The model under review builds one solid part; all positions refer to its coordinate system, in mm. A direction names the side the tool comes from. Give positions to 0.01 mm unless a question says otherwise; leave off trailing zeros. Write each loop counter-clockwise with the first axis right and the second up, starting at its lowest first coordinate (ties: lowest second). Pieces come first, ordered by that corner, then holes. Notation, with made-up numbers: (-39, -12.5) - (4, -12.5) arc R25 cw to (4, 19.5) - close; hole circle Ø11 at (26, 9.25). An arc over 180 degrees is marked (long way). Write item = value, one per line.
```python
from build123d import *

# Parameters (mm, degrees)
SKETCH1_R           = 1.6
SKETCH1_R_2         = 1.75
SKETCH1_R_3         = 3.95
SKETCH1_R_4         = 12
BOSS_EXTRUDE1_DEPTH = 3


with BuildPart() as part:
    # Sketch1 → Boss-Extrude1 (new body)
    with BuildSketch(Plane(origin=(0, 0, 0), x_dir=(1, 0, 0), z_dir=(0, 1, 0))):
        with BuildLine():
            Line((312.373352996, 1022.190294437), (327.907309833, 1022.190294437))
            ThreePointArc((327.907309833, 1022.190294437), (328.157309833, 1022.257281735), (328.340322535, 1022.440294437))
            ThreePointArc((328.340322535, 1022.440294437), (329.126888323, 1022.543848684), (329.023336329, 1021.757282599))
            ThreePointArc((329.023336329, 1021.757282599), (328.840324865, 1021.574270305), (328.773337833, 1021.324271437))
            Line((328.773337833, 1021.324271437), (328.773337833, 1019.690242437))
            ThreePointArc((328.773337833, 1019.690242437), (328.919784442, 1019.336689047), (329.273337833, 1019.190242437))
            Line((329.273337833, 1019.190242437), (334.273335833, 1019.190242437))
            ThreePointArc((334.273335833, 1019.190242437), (334.626889492, 1019.336688397), (334.773336751, 1019.690241519))
            Line((334.773336751, 1019.690241519), (334.773336751, 1021.324268519))
            ThreePointArc((334.773336751, 1021.324268519), (334.706349307, 1021.57426848), (334.523336498, 1021.757281075))
            ThreePointArc((334.523336498, 1021.757281075), (334.419781792, 1022.543846802), (335.206347937, 1022.440295269))
            ThreePointArc((335.206347937, 1022.440295269), (335.389360338, 1022.257283911), (335.639359245, 1022.190297025))
            Line((335.639359245, 1022.190297025), (340.773337745, 1022.190297025))
            Line((340.773337745, 1022.190297025), (340.773337745, 1024.990297025))
            Line((340.773337745, 1024.990297025), (339.423337745, 1024.990297025))
            Line((339.423337745, 1024.990297025), (339.423337745, 1029.190297025))
            Line((339.423337745, 1029.190297025), (340.773337745, 1029.190297025))
            Line((340.773337745, 1029.190297025), (340.773337745, 1032.190297025))
            Line((340.773337745, 1032.190297025), (343.973337745, 1032.190297025))
            Line((343.973337745, 1032.190297025), (343.973337745, 1029.190297025))
            Line((343.973337745, 1029.190297025), (345.323337745, 1029.190297025))
            Line((345.323337745, 1029.190297025), (345.323337745, 1024.990292188))
            Line((345.323337745, 1024.990292188), (343.973337745, 1024.990292188))
            Line((343.973337745, 1024.990292188), (343.973337745, 1022.190292188))
            Line((343.973337745, 1022.190292188), (349.107314245, 1022.190292188))
            ThreePointArc((349.107314245, 1022.190292188), (349.357314245, 1022.257279486), (349.540326947, 1022.440292188))
            ThreePointArc((349.540326947, 1022.440292188), (350.326891976, 1022.543845827), (350.223341741, 1021.75728035))
            ThreePointArc((350.223341741, 1021.75728035), (350.040330277, 1021.574268055), (349.973343245, 1021.324269188))
            Line((349.973343245, 1021.324269188), (349.973343245, 1019.690240188))
            ThreePointArc((349.973343245, 1019.690240188), (350.119789854, 1019.336686797), (350.473343245, 1019.190240188))
            Line((350.473343245, 1019.190240188), (355.473340245, 1019.190240188))
            ThreePointArc((355.473340245, 1019.190240188), (355.826893904, 1019.336686148), (355.973341163, 1019.69023927))
            Line((355.973341163, 1019.69023927), (355.973341163, 1021.32426627))
            ThreePointArc((355.973341163, 1021.32426627), (355.906353816, 1021.574266257), (355.723341079, 1021.757278924))
            ThreePointArc((355.723341079, 1021.757278924), (355.619786681, 1022.543844692), (356.406352785, 1022.44029285))
            ThreePointArc((356.406352785, 1022.44029285), (356.589365548, 1022.257281171), (356.839364996, 1022.190294437))
            Line((356.839364996, 1022.190294437), (372.373340046, 1022.190294437))
            Line((372.373340046, 1022.190294437), (372.373340046, 1072.190301225))
            ThreePointArc((372.373340046, 1072.190301225), (370.908875012, 1075.72583207), (367.373345046, 1077.190299225))
            Line((367.373345046, 1077.190299225), (317.373348046, 1077.190299225))
            ThreePointArc((317.373348046, 1077.190299225), (313.837816014, 1075.725834155), (312.373352996, 1072.190301275))
            Line((312.373352996, 1072.190301275), (312.373352996, 1022.190294437))
        make_face()
        with Locations((366.893344996, 1047.842461747)):
            Circle(SKETCH1_R, mode=Mode.SUBTRACT)
        with Locations((357.873345496, 1071.990299275)):
            Circle(SKETCH1_R_2, mode=Mode.SUBTRACT)
        with Locations((357.873345496, 1040.990299275)):
            Circle(SKETCH1_R_2, mode=Mode.SUBTRACT)
        with Locations((325.373345996, 1051.490299275)):
            Circle(SKETCH1_R_3, mode=Mode.SUBTRACT)
        with Locations((342.373345496, 1056.490299275)):
            Circle(SKETCH1_R_4, mode=Mode.SUBTRACT)
        with Locations((326.873345496, 1071.990299275)):
            Circle(SKETCH1_R_2, mode=Mode.SUBTRACT)
        with Locations((326.873345496, 1040.990299275)):
            Circle(SKETCH1_R_2, mode=Mode.SUBTRACT)
        with Locations((317.853347996, 1047.84952041)):
            Circle(SKETCH1_R, mode=Mode.SUBTRACT)
        with BuildLine():
            Line((365.243389653, 1060.95296097), (365.243389653, 1056.48501097))
            ThreePointArc((365.243389653, 1056.48501097), (365.176400533, 1056.235010504), (364.993385671, 1056.051998658))
            ThreePointArc((364.993385671, 1056.051998658), (364.889836092, 1055.26543287), (365.676401176, 1055.368987799))
            ThreePointArc((365.676401176, 1055.368987799), (365.859413353, 1055.55200075), (366.109412996, 1055.618988627))
            Line((366.109412996, 1055.618988627), (367.677282996, 1055.618988627))
            ThreePointArc((367.677282996, 1055.618988627), (367.927282247, 1055.552001761), (368.110294834, 1055.368990124))
            ThreePointArc((368.110294834, 1055.368990124), (368.896860423, 1055.26543905), (368.793306996, 1056.052004329))
            ThreePointArc((368.793306996, 1056.052004329), (368.610294145, 1056.235017289), (368.543306996, 1056.485017627))
            Line((368.543306996, 1056.485017627), (368.543306996, 1060.952967627))
            ThreePointArc((368.543306996, 1060.952967627), (368.610293862, 1061.202966879), (368.793305499, 1061.385979465))
            ThreePointArc((368.793305499, 1061.385979465), (368.89685718, 1062.172545813), (368.110291294, 1062.068990627))
            ThreePointArc((368.110291294, 1062.068990627), (367.927278767, 1061.885978026), (367.677278996, 1061.818990627))
            Line((367.677278996, 1061.818990627), (366.109410996, 1061.818990627))
            ThreePointArc((366.109410996, 1061.818990627), (365.859411616, 1061.885977015), (365.676398679, 1062.068988302))
            ThreePointArc((365.676398679, 1062.068988302), (364.889832133, 1062.172538478), (364.993388824, 1061.38597279))
            ThreePointArc((364.993388824, 1061.38597279), (365.176401775, 1061.202960613), (365.243389653, 1060.95296097))
        make_face(mode=Mode.SUBTRACT)
        with BuildLine():
            Line((318.637281496, 1061.818997965), (317.069414496, 1061.818997965))
            ThreePointArc((317.069414496, 1061.818997965), (316.819415116, 1061.885984352), (316.636402179, 1062.06899564))
            ThreePointArc((316.636402179, 1062.06899564), (315.849836392, 1062.172545208), (315.953391324, 1061.385980127))
            ThreePointArc((315.953391324, 1061.385980127), (316.136404615, 1061.202967361), (316.203392153, 1060.952966947))
            Line((316.203392153, 1060.952966947), (316.203392153, 1056.485018307))
            ThreePointArc((316.203392153, 1056.485018307), (316.136403033, 1056.235017841), (315.953388171, 1056.052005995))
            ThreePointArc((315.953388171, 1056.052005995), (315.849838592, 1055.265440207), (316.636403676, 1055.368995136))
            ThreePointArc((316.636403676, 1055.368995136), (316.819416286, 1055.552008337), (317.069416496, 1055.618995965))
            Line((317.069416496, 1055.618995965), (318.637286496, 1055.618995965))
            ThreePointArc((318.637286496, 1055.618995965), (318.887285747, 1055.552009098), (319.070298334, 1055.368997461))
            ThreePointArc((319.070298334, 1055.368997461), (319.856863923, 1055.265446387), (319.753310496, 1056.052011666))
            ThreePointArc((319.753310496, 1056.052011666), (319.570297645, 1056.235024626), (319.503310496, 1056.485024964))
            Line((319.503310496, 1056.485024964), (319.503310496, 1060.952974964))
            ThreePointArc((319.503310496, 1060.952974964), (319.570297362, 1061.202974216), (319.753308999, 1061.385986802))
            ThreePointArc((319.753308999, 1061.385986802), (319.85686068, 1062.17255315), (319.070294794, 1062.068997964))
            ThreePointArc((319.070294794, 1062.068997964), (318.887281834, 1061.885985114), (318.637281496, 1061.818997965))
        make_face(mode=Mode.SUBTRACT)
        with BuildLine():
            Line((316.203388653, 1039.193570463), (316.203388653, 1034.725621463))
            ThreePointArc((316.203388653, 1034.725621463), (316.136399531, 1034.475620993), (315.953384663, 1034.292609147))
            ThreePointArc((315.953384663, 1034.292609147), (315.849835095, 1033.506043359), (316.636400176, 1033.609598291))
            ThreePointArc((316.636400176, 1033.609598291), (316.819412786, 1033.792611493), (317.069412996, 1033.85959912))
            Line((317.069412996, 1033.85959912), (318.637282996, 1033.85959912))
            ThreePointArc((318.637282996, 1033.85959912), (318.887282247, 1033.792612254), (319.070294834, 1033.609600616))
            ThreePointArc((319.070294834, 1033.609600616), (319.856860423, 1033.506049543), (319.753306996, 1034.292614822))
            ThreePointArc((319.753306996, 1034.292614822), (319.570294395, 1034.475627349), (319.503306996, 1034.72562712))
            Line((319.503306996, 1034.72562712), (319.503306996, 1039.19357712))
            ThreePointArc((319.503306996, 1039.19357712), (319.570293862, 1039.443576372), (319.753305499, 1039.626588958))
            ThreePointArc((319.753305499, 1039.626588958), (319.856856573, 1040.413154547), (319.070291294, 1040.30960112))
            ThreePointArc((319.070291294, 1040.30960112), (318.887278334, 1040.126588269), (318.637277996, 1040.05960112))
            Line((318.637277996, 1040.05960112), (317.069410996, 1040.05960112))
            ThreePointArc((317.069410996, 1040.05960112), (316.819411616, 1040.126587508), (316.636398679, 1040.309598795))
            ThreePointArc((316.636398679, 1040.309598795), (315.849832892, 1040.413148364), (315.953387824, 1039.626583283))
            ThreePointArc((315.953387824, 1039.626583283), (316.136401025, 1039.443570673), (316.203388653, 1039.193570463))
        make_face(mode=Mode.SUBTRACT)
        with BuildLine():
            Line((368.543303996, 1034.72562712), (368.543303996, 1039.19357712))
            ThreePointArc((368.543303996, 1039.19357712), (368.610290862, 1039.443576372), (368.793302499, 1039.626588958))
            ThreePointArc((368.793302499, 1039.626588958), (368.896853573, 1040.413154547), (368.110288294, 1040.30960112))
            ThreePointArc((368.110288294, 1040.30960112), (367.927275767, 1040.126588519), (367.677275996, 1040.05960112))
            Line((367.677275996, 1040.05960112), (366.109407996, 1040.05960112))
            ThreePointArc((366.109407996, 1040.05960112), (365.859408616, 1040.126587508), (365.676395679, 1040.309598795))
            ThreePointArc((365.676395679, 1040.309598795), (364.889829133, 1040.413148971), (364.993385824, 1039.626583283))
            ThreePointArc((364.993385824, 1039.626583283), (365.176399025, 1039.443570673), (365.243386653, 1039.193570463))
            Line((365.243386653, 1039.193570463), (365.243386653, 1034.725621463))
            ThreePointArc((365.243386653, 1034.725621463), (365.176397531, 1034.475620993), (364.993382663, 1034.292609147))
            ThreePointArc((364.993382663, 1034.292609147), (364.889833095, 1033.506043359), (365.676398176, 1033.609598291))
            ThreePointArc((365.676398176, 1033.609598291), (365.859410353, 1033.792611243), (366.109409996, 1033.85959912))
            Line((366.109409996, 1033.85959912), (367.677279996, 1033.85959912))
            ThreePointArc((367.677279996, 1033.85959912), (367.927279247, 1033.792612254), (368.110291834, 1033.609600616))
            ThreePointArc((368.110291834, 1033.609600616), (368.896857423, 1033.506049543), (368.793303996, 1034.292614822))
            ThreePointArc((368.793303996, 1034.292614822), (368.610291395, 1034.475627349), (368.543303996, 1034.72562712))
        make_face(mode=Mode.SUBTRACT)
    extrude(amount=BOSS_EXTRUDE1_DEPTH)


solid = part.part
```
1. Machinability: for faces 3 (the flat face through (316.203, 1, -1037)), 4 (the flat face through (372.373, 1, -1047)), 5 (the flat face through (334.773, 1, -1020)), which of the approach directions +Z, -Z, +X, -X, +Y, -Y give a long, thin tool a straight path to every point of the face, cutting with its end or side? Answer none if there is none.
Findings below:
face_3 = +Y, -Y
face_4 = +Z, -Z, +X, +Y, -Y
face_5 = +Z, +Y, -Y
2. Take a section at C-C on x = 347. Give the boundary of the cut face in (y, z), and give its area (3 significant figures).
Findings below:
outline = (0, -1077.19) - (3, -1077.19) - (3, -1067.56) - (0, -1067.56) - close; (0, -1045.42) - (3, -1045.42) - (3, -1022.19) - (0, -1022.19) - close
area = 98.6 mm²
3. For line 1 (X direction, y = 0.9, z = -1036.5); line 2 (Z direction, x = 319, y = 2.9); line 3 (X direction, y = 2.7, z = -1049), list the stretches that pass through material, from the lowest coordinate up. Write a range as from..to.
Findings below:
line_1 = 312.37..316.2, 319.5..365.24, 368.54..372.37
line_2 = -1077.19..-1061.97, -1055.46..-1048.97, -1046.73..-1040.22, -1033.7..-1022.19
line_3 = 312.37..316.74, 318.97..322.31, 328.44..333, 351.75..365.79, 368..372.37
4. Take a section at A-A on z = -1027. Give the boundary of the cut face in (x, y), and give its area (3 significant figures).
Findings below:
outline = (312.37, 0) - (339.42, 0) - (339.42, 3) - (312.37, 3) - close; (345.32, 0) - (372.37, 0) - (372.37, 3) - (345.32, 3) - close
area = 162 mm²
5. Insertion check: P1, Ø1.1, axis at x = 340.5, y = 1, coming from the +Z side; P2, Ø6.5, axis at x = 325.37, z = -1051.49, coming from the +Y side; P3, Ø0.5, axis at y = 2, z = -1020.5, coming from the -X side. Each pin has a flat end and moves straight along its axis. Give the tip position at first contact, or say it passes through.
Findings below:
P1 = -1022.19
P2 = through
P3 = 328.77
6. Take a section at B-B on x = 326. Give the boundary of the cut face in (y, z).
Findings below:
outline = (0, -1077.19) - (3, -1077.19) - (3, -1073.51) - (0, -1073.51) - close; (0, -1070.47) - (3, -1070.47) - (3, -1055.39) - (0, -1055.39) - close; (0, -1047.59) - (3, -1047.59) - (3, -1042.51) - (0, -1042.51) - close; (0, -1039.47) - (3, -1039.47) - (3, -1022.19) - (0, -1022.19) - close
7. Take a section at D-D on y = 0.65. Count the separate pieces of the cut face and the enclosed holes in it, and give its area (3 significant figures).
Findings below:
separate_pieces = 1
enclosed_holes = 12
area = 2,630 mm²
8. Draft analysis for pull direction Z (two halves, no side actions). For faces 1 (the cylindrical face through (316.255, 1.479, -1047.92)), 2 (the flat face through (340.773, 1, -1031)), state which applies: +Z half, -Z half, draft (parallel to the pull), parting line (faces both ways), or undercut.
Findings below:
face_1 = undercut
face_2 = draft
